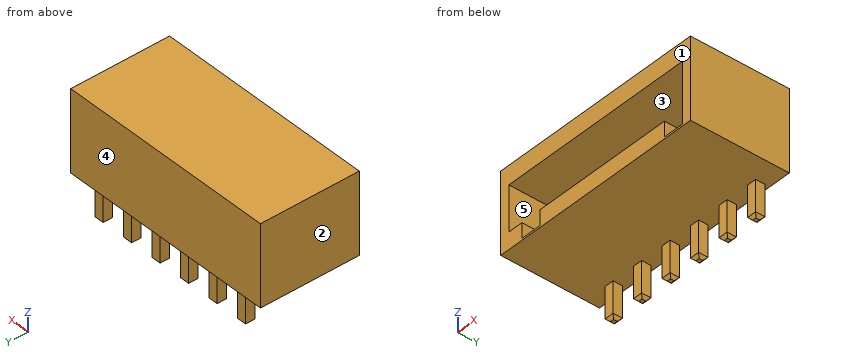
```python
from build123d import *

# Parameters (mm, degrees)
SKETCH_1_W                         = 23.3
SKETCH_1_H                         = 10.5
EXTRUDE_1_DEPTH                    = 8.6
CUT_EXTRUDE_1_DEPTH                = 7
EXTRUDE_START                      = -5
SKETCH_3_W                         = 1
SKETCH_3_H                         = 1
EXTRUDE_2_DEPTH                    = 8.6
CHAMFER_1_SIZE                     = 0.3
PATTERN_LINEAR_1_COUNT             = 6
PATTERN_LINEAR_1_PITCH             = 3.5
CHAMFER_1_OF_PATTERN_LINEAR_1_SIZE = 0.3


with BuildPart() as part:
    # Эскиз1 → Бобышка-Вытянуть1 (new body)
    with BuildSketch(Plane.XY):
        Rectangle(SKETCH_1_W, SKETCH_1_H)
    extrude(amount=EXTRUDE_1_DEPTH)

    # Эскиз2 → Вырез-Вытянуть1 (cut)
    with BuildSketch(Plane.XZ.offset(5.25)):
        Polygon((-10.65, 6.6), (10.65, 6.6), (10.65, 0.2), (8.45, 0.2), (8.45, 1.8), (-6.85, 1.8), (-6.85, 0.2), (-9.05, 0.2), (-9.05, 1.8), (-10.65, 1.8), align=None)
    extrude(amount=-CUT_EXTRUDE_1_DEPTH, mode=Mode.SUBTRACT)

    # Эскиз3 → Бобышка-Вытянуть2 (add)
    with BuildSketch(Plane(origin=(0, 0, 0), x_dir=(-1, 0, 0), z_dir=(0, 0, -1)).offset(EXTRUDE_START)):
        with Locations((8.75, 4.25)):
            Rectangle(SKETCH_3_W, SKETCH_3_H)
    extrude_2 = extrude(amount=EXTRUDE_2_DEPTH)

    # Фаска1
    chamfer_1_edges = [part.edges().sort_by_distance(p)[0] for p in [
        (-8.25, 4.25, -3.6),
        (-8.75, 3.75, -3.6),
        (-9.25, 4.25, -3.6),
        (-8.75, 4.75, -3.6),
    ]]
    chamfer(chamfer_1_edges, length=CHAMFER_1_SIZE)

    # Линейный массив1: Бобышка-Вытянуть2 ×6
    with Locations(*[(i * PATTERN_LINEAR_1_PITCH, 0, 0) for i in range(1, PATTERN_LINEAR_1_COUNT)]):
        add(extrude_2)

    # Фаска1 of Линейный массив1
    chamfer_1_of_pattern_linear_1_edges = [part.edges().sort_by_distance(p)[0] for p in [
        (-4.75, 4.25, -3.6),
        (-5.25, 3.75, -3.6),
        (-5.75, 4.25, -3.6),
        (-5.25, 4.75, -3.6),
        (-1.25, 4.25, -3.6),
        (-1.75, 3.75, -3.6),
        (-2.25, 4.25, -3.6),
        (-1.75, 4.75, -3.6),
        (2.25, 4.25, -3.6),
        (1.75, 3.75, -3.6),
        (1.25, 4.25, -3.6),
        (1.75, 4.75, -3.6),
        (5.75, 4.25, -3.6),
        (5.25, 3.75, -3.6),
        (4.75, 4.25, -3.6),
        (5.25, 4.75, -3.6),
        (9.25, 4.25, -3.6),
        (8.75, 3.75, -3.6),
        (8.25, 4.25, -3.6),
        (8.75, 4.75, -3.6),
    ]]
    chamfer(chamfer_1_of_pattern_linear_1_edges, length=CHAMFER_1_OF_PATTERN_LINEAR_1_SIZE)


solid = part.part
```
Input: part model. Units: mm. Frame: model coordinates. Face numbers are marked on the shaded views. A direction names the side the tool comes from. Give positions to 0.01 mm unless a question says otherwise; leave off trailing zeros. Order: outer loops, then holes, each group sorted by start corner. A loop starts at its lowest first (then second) coordinate and runs counter-clockwise, first axis right, second up. Notation, with made-up numbers: (83, -36.5) - (110, -36.5) arc R24 ccw to (110, -5.5) - close; hole circle Ø11 at (44.5, 28). An arc over 180 degrees is marked (long way). One line per item, written item: value.
1. Draft query along X for the marked faces 1, 2 and 3. Return one class per face: released by +X, released by -X, zero draft, split by the parting line, or undercut.
Determined:
face 1: zero draft
face 2: released by -X
face 3: undercut
2. Reachability of the marked faces 4 and 5 from +Z, -Z, +X, -X, +Y, -Y: full face, straight path, thin tool, end or side. Return the list, or none.
Determined:
face 4: +Z, -Z, +X, -X, +Y
face 5: -Y
3. Pin query (flat end, axial travel): pin 1 Ø0.8 at (x, z) = (5.5, -2.5) entering from +Y; pin 2 Ø0.5 at (x, z) = (-5, -1) entering from -Y; pin 3 Ø1.5 at (x, z) = (-5.5, -2) entering from -Y. Return the tip coordinate at first contact, or that it passes through.
Determined:
pin 1: y = 4.75
pin 2: y = 3.75
pin 3: y = 3.75
4. Cut plane D-D, the plane z = 5.75. Output: boundary loops of the cut face in (x, y).
Determined:
outline: (-11.65, -5.25) - (-10.65, -5.25) - (-10.65, 1.75) - (10.65, 1.75) - (10.65, -5.25) - (11.65, -5.25) - (11.65, 5.25) - (-11.65, 5.25) - close
5. Line query: probe 1 along X at (y, z) = (-3.75, 0.75); probe 2 along X at (y, z) = (0.5, 3.5); probe 3 along Z at (x, y) = (-4.75, -4.5). Output: solid intervals per line, ascending.
Determined:
probe 1: -11.65 to -9.05, -6.85 to 8.45, 10.65 to 11.65
probe 2: -11.65 to -10.65, 10.65 to 11.65
probe 3: 0 to 1.8, 6.6 to 8.6
6. Cut plane B-B, the plane z = -2.25. Output: boundary loops of the cut face in (x, y).
Determined:
outline: (-9.25, 3.75) - (-8.25, 3.75) - (-8.25, 4.75) - (-9.25, 4.75) - close; (-5.75, 3.75) - (-4.75, 3.75) - (-4.75, 4.75) - (-5.75, 4.75) - close; (-2.25, 3.75) - (-1.25, 3.75) - (-1.25, 4.75) - (-2.25, 4.75) - close; (1.25, 3.75) - (2.25, 3.75) - (2.25, 4.75) - (1.25, 4.75) - close; (4.75, 3.75) - (5.75, 3.75) - (5.75, 4.75) - (4.75, 4.75) - close; (8.25, 3.75) - (9.25, 3.75) - (9.25, 4.75) - (8.25, 4.75) - close
7. Cut plane A-A, the plane y = 1.25. Output: boundary loops of the cut face in (x, z), and give its area (3 significant figures).
Determined:
outline: (-11.65, 0) - (11.65, 0) - (11.65, 8.6) - (-11.65, 8.6) - close; hole (-10.65, 1.8) - (-9.05, 1.8) - (-9.05, 0.2) - (-6.85, 0.2) - (-6.85, 1.8) - (8.45, 1.8) - (8.45, 0.2) - (10.65, 0.2) - (10.65, 6.6) - (-10.65, 6.6) - close
area: 91.1 mm2
8. Cut plane C-C, the plane x = -3.5. Output: boundary loops of the cut face in (y, z), and give its area (3 significant figures).
Determined:
outline: (-5.25, 0) - (5.25, 0) - (5.25, 8.6) - (-5.25, 8.6) - (-5.25, 6.6) - (1.75, 6.6) - (1.75, 1.8) - (-5.25, 1.8) - close
area: 56.7 mm2
